from build123d import *

# Parameters (mm, degrees)
SKETCH_1_R      = 1.6
SKETCH_1_R_2    = 13.6
EXTRUDE_1_DEPTH = 8
FILLET_1_R      = 4


with BuildPart() as part:
    # Sketch 1 → Extrude 1 (new body)
    with BuildSketch(Plane(origin=(0, 0, 0), x_dir=(1, 0, 0), z_dir=(0, 1, 0))):
        with BuildLine():
            ThreePointArc((17.042857143, -3.973791692), (21.5, 0), (17.042857143, 3.973791692))
            ThreePointArc((17.042857143, 3.973791692), (12.374368671, 12.374368671), (3.973791692, 17.042857143))
            ThreePointArc((3.973791692, 17.042857143), (0, 21.5), (-3.973791692, 17.042857143))
            ThreePointArc((-3.973791692, 17.042857143), (-12.374368671, 12.374368671), (-17.042857143, 3.973791692))
            ThreePointArc((-17.042857143, 3.973791692), (-21.5, 0), (-17.042857143, -3.973791692))
            ThreePointArc((-17.042857143, -3.973791692), (-12.374368671, -12.374368671), (-3.973791692, -17.042857143))
            ThreePointArc((-3.973791692, -17.042857143), (0, -21.5), (3.973791692, -17.042857143))
            ThreePointArc((3.973791692, -17.042857143), (12.374368671, -12.374368671), (17.042857143, -3.973791692))
        make_face()
        with Locations(Location((17.5, 0, 0), (0, 0, 270))):
            Circle(SKETCH_1_R, mode=Mode.SUBTRACT)
        with Locations(Location((-17.5, 0, 0), (0, 0, 270))):
            Circle(SKETCH_1_R, mode=Mode.SUBTRACT)
        with Locations(Location((0, 0, 0), (0, 0, 270))):
            Circle(SKETCH_1_R_2, mode=Mode.SUBTRACT)
        with Locations(Location((0, 17.5, 0), (0, 0, 270))):
            Circle(SKETCH_1_R, mode=Mode.SUBTRACT)
        with Locations(Location((0, -17.5, 0), (0, 0, 270))):
            Circle(SKETCH_1_R, mode=Mode.SUBTRACT)
    extrude(amount=EXTRUDE_1_DEPTH)

    # Fillet 1
    fillet_1_edges = [part.edges().sort_by_distance(p)[0] for p in [
        (17.042857143, 4, 3.973791692),
        (3.973791692, 4, 17.042857143),
        (-3.973791692, 4, 17.042857143),
        (-17.042857143, 4, 3.973791692),
        (-17.042857143, 4, -3.973791692),
        (-3.973791692, 4, -17.042857143),
        (3.973791692, 4, -17.042857143),
        (17.042857143, 4, -3.973791692),
    ]]
    fillet(fillet_1_edges, radius=FILLET_1_R)


solid = part.part
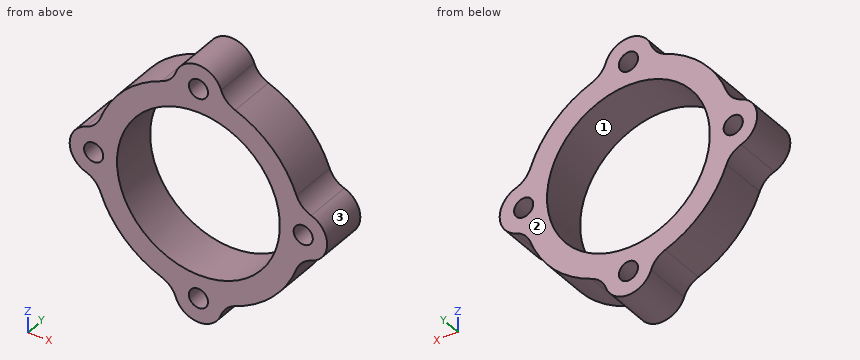
Design review of the part built by this model. Coordinates are the model's own, in mm. Face numbers are marked on the shaded views. Coordinates: 2 decimals unless noted, no trailing zeros. Loops run counter-clockwise (first coordinate to the right, second up) from the corner with the lowest first, then second, coordinate; pieces in that order, holes last. Notation, with made-up numbers: (9.25, -39) -> (48.25, -39) arc R29 cw to (48.25, -9) -> close; hole circle Ø2 at (-34.75, 75). An arc over 180 degrees is marked (long way). Use a Markdown table: item, result. Add a question column.
Item 1: Clearance check with flat-ended pins moving along their axes: P1, Ø1.9, axis at x = 17.5, z = 0, coming from the -Y side; P2, Ø1.5, axis at y = 6, z = 1, coming from the +X side; P3, Ø1.5, axis at x = -15.5, y = 1.5, coming from the -Z side. State where each tip first meets the part, or that it passes through.
Item 2: We need section D-D, the plane y = 4.75. Count the separate pieces of the cut face and the enclosed holes in it, and give its area (3 significant figures).
Item 3: We need section A-A, the plane z = 0. Write out the cut boundary in (x, y).
Item 4: The part is to be moulded in two halves that separate along Z. For the marked faces 1, 2 and 3, say which applies: +Z half, -Z half, draft (parallel to the pull), parting line (faces both ways), or undercut.
Item 5: We need section C-C, the plane z = -13. Write out the cut boundary in (x, y) (3 decimals), and give its area (3 significant figures).
Item 6: Wall thickness on L1, parallel to X at y = 3.5, z = 0; L2, parallel to X at y = 3.5, z = -1; L3, parallel to X at y = 6, z = -7: over which ranges is each line inside the solid? List them lowest first. Write a range as from..to.
Item 7: We need section B-B, the plane x = -10. Write out the cut boundary in (y, z).
Numbers:
| question | item | result |
|---|---|---|
| 1 | P1 | passes through |
| 1 | P2 | stops at x = 21.49 |
| 1 | P3 | stops at z = -9.42 |
| 2 | separate pieces | 1 |
| 2 | enclosed holes | 5 |
| 2 | area | 461 mm^2 |
| 3 | outline | (-21.5, 0) -> (-19.1, 0) -> (-19.1, 8) -> (-21.5, 8) -> close; (-15.9, 0) -> (-13.6, 0) -> (-13.6, 8) -> (-15.9, 8) -> close; (13.6, 0) -> (15.9, 0) -> (15.9, 8) -> (13.6, 8) -> close; (19.1, 0) -> (21.5, 0) -> (21.5, 8) -> (19.1, 8) -> close |
| 4 | face 1 | undercut |
| 4 | face 2 | draft |
| 4 | face 3 | parting line |
| 5 | outline | (-11.715, 0) -> (-3.995, 0) -> (-3.995, 8) -> (-11.715, 8) -> close; (3.995, 0) -> (11.715, 0) -> (11.715, 8) -> (3.995, 8) -> close |
| 5 | area | 124 mm^2 |
| 6 | L1 | x = -21.5..-19.1, -15.9..-13.6, 13.6..15.9, 19.1..21.5 |
| 6 | L2 | x = -21.37..-18.75, -16.25..-13.56, 13.56..16.25, 18.75..21.37 |
| 6 | L3 | x = -16.04..-11.66, 11.66..16.04 |
| 7 | outline | (0, -14.36) -> (8, -14.36) -> (8, -9.22) -> (0, -9.22) -> close; (0, 9.22) -> (8, 9.22) -> (8, 14.36) -> (0, 14.36) -> close |
